from build123d import *

# Parameters (mm, degrees)
SKETCH1_W           = 20
SKETCH1_H           = 5
BOSS_EXTRUDE1_DEPTH = 4
BOSS_EXTRUDE2_DEPTH = 2
CHAMFER1_SIZE       = 0.5
CHAMFER2_SIZE       = 1
CHAMFER3_SIZE       = 1
CHAMFER3_SIZE2      = 0.707106781
FILLET5_R           = 1


with BuildPart() as part:
    # Sketch1 → Boss-Extrude1 (new body)
    with BuildSketch(Plane.XY):
        Polygon((-15, 7.5), (-15, -7.5), (-10, -2.5), (-10, 2.5), align=None)
        Rectangle(SKETCH1_W, SKETCH1_H)
        Polygon((10, 2.5), (15, 7.5), (15, -7.5), (10, -2.5), align=None)
    extrude(amount=BOSS_EXTRUDE1_DEPTH)

    # Sketch4 → Boss-Extrude2 (add, symmetric)
    with BuildSketch(Plane(origin=(0, 0, 0), x_dir=(1, 0, 0), z_dir=(0, 1, 0))):
        Polygon((3.5, 0), (-8.5, 7), (-8.5, 5), (-3.5, 0), align=None)
    extrude(amount=BOSS_EXTRUDE2_DEPTH, both=True)

    # Chamfer1
    chamfer1_edges = [part.edges().sort_by_distance(p)[0] for p in [
        (-12.5, -5, 4),
        (0, -2.5, 4),
        (12.5, -5, 4),
        (15, 0, 4),
        (12.5, 5, 4),
        (0, 2.5, 4),
        (-12.5, 5, 4),
        (-15, 0, 4),
    ]]
    chamfer(chamfer1_edges, length=CHAMFER1_SIZE)

    # Chamfer2
    # the kernel refuses this chamfer: 1 mm, written as the material it takes off along each edge
    with BuildSketch(Plane(origin=(16.81845448, -9.31845448, 0), x_dir=(0.7071067811865414, 0.7071067811865538, 0), z_dir=(-0.7071067811865538, 0.7071067811865415, 0))) as chamfer2_piece_1_section:
        Polygon((CHAMFER2_SIZE, 0), (0, -CHAMFER2_SIZE), (0, 0), align=None)
    chamfer2_piece_1 = extrude(amount=12.214433788, mode=Mode.PRIVATE)
    chamfer2_piece_1 = split(chamfer2_piece_1, bisect_by=Plane(origin=(16.81845448, -5.40922724, 3.90922724), z_dir=(0, -0.7071067811865476, -0.7071067811865476)), keep=Keep.TOP, mode=Mode.PRIVATE)
    add(chamfer2_piece_1, mode=Mode.SUBTRACT)
    with BuildSketch(Plane(origin=(15, 10.071682988, 0), x_dir=(-1, 0, 0), z_dir=(0, -1, 0)), Plane(origin=(-15, 10.071682988, 0), x_dir=(0, 0, 1), z_dir=(0, -1, 0))) as chamfer2_piece_2:
        Polygon((CHAMFER2_SIZE, 0), (0, -CHAMFER2_SIZE), (0, 0), align=None)
    extrude(amount=20.143365976, mode=Mode.SUBTRACT)
    with BuildSketch(Plane(origin=(8.18154552, 0.68154552, 0), x_dir=(0.707106781186537, -0.7071067811865581, 0), z_dir=(0.7071067811865581, 0.707106781186537, 0))) as chamfer2_piece_3_section:
        Polygon((CHAMFER2_SIZE, 0), (0, -CHAMFER2_SIZE), (0, 0), align=None)
    chamfer2_piece_3 = extrude(amount=12.214433788, mode=Mode.PRIVATE)
    chamfer2_piece_3 = split(chamfer2_piece_3, bisect_by=Plane(origin=(8.18154552, 1.09077276, -0.40922724), z_dir=(0, 0.7071067811865476, -0.7071067811865476)), keep=Keep.TOP, mode=Mode.PRIVATE)
    add(chamfer2_piece_3, mode=Mode.SUBTRACT)
    with BuildSketch(Plane(origin=(12.571682988, 2.5, 0), x_dir=(0, -1, 0), z_dir=(-1, 0, 0))) as chamfer2_piece_4_section:
        Polygon((CHAMFER2_SIZE, 0), (0, CHAMFER2_SIZE), (0, 0), align=None)
    chamfer2_piece_4 = extrude(amount=25.143365976, mode=Mode.PRIVATE)
    chamfer2_piece_4 = split(chamfer2_piece_4, bisect_by=Plane(origin=(10.268509587, 2.5, 3.948297259), z_dir=(0.5038710255240867, 0, -0.8637789008984332)), keep=Keep.TOP, mode=Mode.PRIVATE)
    chamfer2_piece_4 = split(chamfer2_piece_4, bisect_by=Plane(origin=(12.282315632, 2.789367356, -0.40922724), z_dir=(-0.4999999999999927, 0.5000000000000075, -0.7071067811865475)), keep=Keep.TOP, mode=Mode.PRIVATE)
    add(chamfer2_piece_4, mode=Mode.SUBTRACT)
    with BuildSketch(Plane(origin=(12.571682988, 2.5, 0), x_dir=(0, -1, 0), z_dir=(-1, 0, 0))) as chamfer2_piece_5_section:
        Polygon((CHAMFER2_SIZE, 0), (0, CHAMFER2_SIZE), (0, 0), align=None)
    chamfer2_piece_5 = extrude(amount=25.143365976, mode=Mode.PRIVATE)
    chamfer2_piece_5 = split(chamfer2_piece_5, bisect_by=Plane(origin=(12.571682988, 2, 0), z_dir=(0, 1, 0)), keep=Keep.TOP, mode=Mode.PRIVATE)
    chamfer2_piece_5 = split(chamfer2_piece_5, bisect_by=Plane(origin=(12.282315632, 2.789367356, -0.40922724), z_dir=(-0.4999999999999927, 0.5000000000000075, -0.7071067811865475)), keep=Keep.TOP, mode=Mode.PRIVATE)
    chamfer2_piece_5 = split(chamfer2_piece_5, bisect_by=Plane(origin=(6.57520885, -3.496474138, 8.480295052), z_dir=(0.49999999999999395, 0.500000000000006, -0.7071067811865475)), keep=Keep.TOP, mode=Mode.PRIVATE)
    add(chamfer2_piece_5, mode=Mode.SUBTRACT)
    with BuildSketch(Plane(origin=(12.571682988, 2.5, 0), x_dir=(0, -1, 0), z_dir=(-1, 0, 0))) as chamfer2_piece_6_section:
        Polygon((CHAMFER2_SIZE, 0), (0, CHAMFER2_SIZE), (0, 0), align=None)
    chamfer2_piece_6 = extrude(amount=25.143365976, mode=Mode.PRIVATE)
    chamfer2_piece_6 = split(chamfer2_piece_6, bisect_by=Plane(origin=(4.535841494, 2.5, 8.035841494), z_dir=(-0.7071067811865487, 0, 0.7071067811865464)), keep=Keep.TOP, mode=Mode.PRIVATE)
    chamfer2_piece_6 = split(chamfer2_piece_6, bisect_by=Plane(origin=(6.57520885, -3.496474138, 8.480295052), z_dir=(0.49999999999999395, 0.500000000000006, -0.7071067811865475)), keep=Keep.TOP, mode=Mode.PRIVATE)
    add(chamfer2_piece_6, mode=Mode.SUBTRACT)
    with BuildSketch(Plane(origin=(-12.571682988, -2.5, 0), x_dir=(0, 1, 0), z_dir=(1, 0, 0))) as chamfer2_piece_7_section:
        Polygon((CHAMFER2_SIZE, 0), (0, CHAMFER2_SIZE), (0, 0), align=None)
    chamfer2_piece_7 = extrude(amount=25.143365976, mode=Mode.PRIVATE)
    chamfer2_piece_7 = split(chamfer2_piece_7, bisect_by=Plane(origin=(-8.035841494, -2.5, -4.535841494), z_dir=(-0.7071067811865487, 0, 0.7071067811865464)), keep=Keep.TOP, mode=Mode.PRIVATE)
    chamfer2_piece_7 = split(chamfer2_piece_7, bisect_by=Plane(origin=(-12.282315632, -2.789367356, -0.40922724), z_dir=(0.499999999999994, -0.5000000000000063, -0.7071067811865475)), keep=Keep.TOP, mode=Mode.PRIVATE)
    add(chamfer2_piece_7, mode=Mode.SUBTRACT)
    with BuildSketch(Plane(origin=(-12.571682988, -2.5, 0), x_dir=(0, 1, 0), z_dir=(1, 0, 0))) as chamfer2_piece_8_section:
        Polygon((CHAMFER2_SIZE, 0), (0, CHAMFER2_SIZE), (0, 0), align=None)
    chamfer2_piece_8 = extrude(amount=25.143365976, mode=Mode.PRIVATE)
    chamfer2_piece_8 = split(chamfer2_piece_8, bisect_by=Plane(origin=(-12.571682988, -2, 0), z_dir=(0, -1, 0)), keep=Keep.TOP, mode=Mode.PRIVATE)
    chamfer2_piece_8 = split(chamfer2_piece_8, bisect_by=Plane(origin=(-12.282315632, -2.789367356, -0.40922724), z_dir=(0.499999999999994, -0.5000000000000063, -0.7071067811865475)), keep=Keep.TOP, mode=Mode.PRIVATE)
    chamfer2_piece_8 = split(chamfer2_piece_8, bisect_by=Plane(origin=(-6.57520885, 3.496474138, 8.480295052), z_dir=(-0.49999999999999584, -0.5000000000000047, -0.7071067811865475)), keep=Keep.TOP, mode=Mode.PRIVATE)
    add(chamfer2_piece_8, mode=Mode.SUBTRACT)
    with BuildSketch(Plane(origin=(-12.571682988, -2.5, 0), x_dir=(0, 1, 0), z_dir=(1, 0, 0))) as chamfer2_piece_9_section:
        Polygon((CHAMFER2_SIZE, 0), (0, CHAMFER2_SIZE), (0, 0), align=None)
    chamfer2_piece_9 = extrude(amount=25.143365976, mode=Mode.PRIVATE)
    chamfer2_piece_9 = split(chamfer2_piece_9, bisect_by=Plane(origin=(-8.491307514, -2.5, -6.994929383), z_dir=(0.5038710255240867, 0, -0.8637789008984332)), keep=Keep.TOP, mode=Mode.PRIVATE)
    chamfer2_piece_9 = split(chamfer2_piece_9, bisect_by=Plane(origin=(-6.57520885, 3.496474138, 8.480295052), z_dir=(-0.49999999999999584, -0.5000000000000047, -0.7071067811865475)), keep=Keep.TOP, mode=Mode.PRIVATE)
    add(chamfer2_piece_9, mode=Mode.SUBTRACT)
    with BuildSketch(Plane(origin=(-16.81845448, -9.31845448, 0), x_dir=(-0.7071067811865389, 0.7071067811865562, 0), z_dir=(0.7071067811865562, 0.7071067811865389, 0))) as chamfer2_piece_10_section:
        Polygon((CHAMFER2_SIZE, 0), (0, CHAMFER2_SIZE), (0, 0), align=None)
    chamfer2_piece_10 = extrude(amount=12.214433788, mode=Mode.PRIVATE)
    chamfer2_piece_10 = split(chamfer2_piece_10, bisect_by=Plane(origin=(-16.81845448, -5.40922724, 3.90922724), z_dir=(0, -0.7071067811865476, -0.7071067811865476)), keep=Keep.TOP, mode=Mode.PRIVATE)
    add(chamfer2_piece_10, mode=Mode.SUBTRACT)
    with BuildSketch(Plane(origin=(-8.18154552, 0.68154552, 0), x_dir=(0, 0, 1), z_dir=(-0.707106781186556, 0.707106781186539, 0))) as chamfer2_piece_11_section:
        Polygon((CHAMFER2_SIZE, 0), (0, -CHAMFER2_SIZE), (0, 0), align=None)
    chamfer2_piece_11 = extrude(amount=12.214433788, mode=Mode.PRIVATE)
    chamfer2_piece_11 = split(chamfer2_piece_11, bisect_by=Plane(origin=(-8.18154552, 1.09077276, -0.40922724), z_dir=(0, 0.7071067811865476, -0.7071067811865476)), keep=Keep.TOP, mode=Mode.PRIVATE)
    add(chamfer2_piece_11, mode=Mode.SUBTRACT)

    # Chamfer3
    chamfer3_edges = [part.edges().sort_by_distance(p)[0] for p in [
        (-3.5, 0, 0),
    ]]
    chamfer3_side = [part.faces().sort_by_distance(p)[0] for p in [
        (-5.967078189, 0, -2.467078189),
    ]]
    chamfer(chamfer3_edges, length=CHAMFER3_SIZE, length2=CHAMFER3_SIZE2, reference=chamfer3_side[0])

    # Fillet5
    # the kernel refuses this fillet: 1 mm, written as the material it takes off along each edge
    with BuildSketch(Plane(origin=(-8.5, -6.352592498, -7), x_dir=(0, 0, 1), z_dir=(0, 1, 0))) as fillet5_piece_1:
        with BuildLine():
            CenterArc((FILLET5_R * 1.74103699912, FILLET5_R), FILLET5_R, 149.743562836, 120.256437164)
            Line((FILLET5_R * 0.877258098223, FILLET5_R * 1.50387102552), (0, 0))
            Line((0, 0), (FILLET5_R * 1.74103699912, 0))
        make_face()
    extrude(amount=12.705184996, mode=Mode.SUBTRACT)
    with BuildSketch(Plane(origin=(-8.5, -3.035533906, -5), x_dir=(0, 0, -1), z_dir=(0, 1, 0))) as fillet5_piece_2:
        with BuildLine():
            CenterArc((FILLET5_R * 0.414213562373, -FILLET5_R), FILLET5_R, 90, 45)
            Line((-FILLET5_R * 0.292893218813, -FILLET5_R * 0.292893218813), (0, 0))
            Line((0, 0), (FILLET5_R * 0.414213562373, 0))
        make_face()
    extrude(amount=6.071067812, mode=Mode.SUBTRACT)


solid = part.part
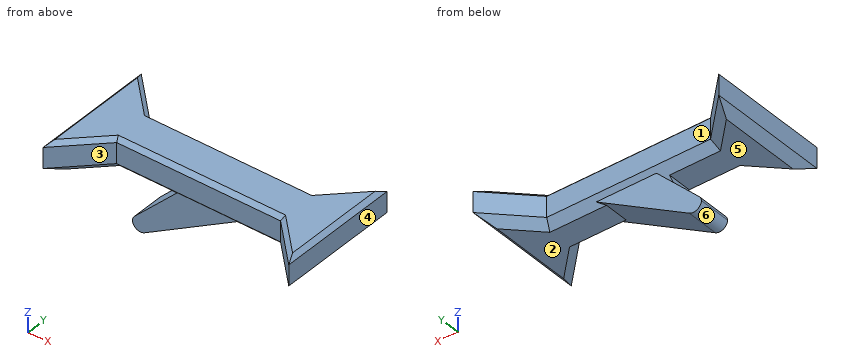
Geometry check sheet. Reference: the model listing, model coordinates, mm. Face numbers are marked on the shaded views. A direction names the side the tool comes from. Give positions to 0.01 mm unless a question says otherwise; leave off trailing zeros. Write each loop counter-clockwise with the first axis right and the second up, starting at its lowest first coordinate (ties: lowest second). Pieces come first, ordered by that corner, then holes. Notation, with made-up numbers: M 39,13.25 L 81,13.25 A31 cw 81,40.25 Z; hole C 45.25,42 d1. An arc over 180 degrees is marked long. Answer as CSV lines item,"result". Start each with the question number.
Q1. Section check C-C, the plane y = 3. Record the cut outline in (x, z), then the cut area to 3 significant figures.
Q2. Section check A-A, the plane x = -5.5. Record the cut outline in (y, z), then the cut area to 4 significant figures.
Q3. Release check for a two-part mould opening along Z. For the marked faces 4, 5 and 6 record: pulls with the +Z half, pulls with the -Z half, needs draft (parallel to the pull), parting line crosses it, or undercut.
Q4. Section check B-B, the plane z = 2.75. Record the cut outline in (x, y), then the cut area to 3 significant figures.
Q5. Section check D-D, the plane x = 5. Record the cut outline in (y, z).
Q6. Tool access check on the marked faces 1, 2 and 3. Record the directions out of +Z, -Z, +X, -X, +Y, -Y that give a thin tool (end or side, any length) a straight path to the whole face; none if there is none.
Q7. Material ranges on L1, parallel to Y at x = -6.5, z = -4; L2, parallel to Y at x = 3.5, z = 1.75; L3, parallel to X at y = -4, z = 0.75, recorded low to high.
Q8. Go/stop test with flat-tipped pins: pin 1 (5 mm diameter, centred on x = 3, z = 0, fed in from +Y); pin 2 (0.8 mm diameter, centred on x = -2, z = 2.5, fed in from -Y); pin 3 (5 mm diameter, centred on x = 11.5, y = 3.5, fed in from -Z). Record where each tip stops, or that it passes through.
Geometry says:
1,outline,"M -15,1 L -14,0 L -11.91,0 L -10.5,1 L -10.5,3.5 L -11.21,4 L -14.5,4 L -15,3.5 Z; M 10.5,1 L 11.91,0 L 14,0 L 15,1 L 15,3.5 L 14.5,4 L 11.21,4 L 10.5,3.5 Z"
1,area,"33.0 mm^2"
2,outline,"M -2.5,1 L -1.5,0 L 1.5,0 L 2.5,1 L 2.5,3.5 L 2,4 L -2,4 L -2.5,3.5 Z; M -2,-5.25 L 2,-5.25 L 2,-2 L -2,-2 Z"
2,area,"31.75 mm^2"
3,face 4,"needs draft"
3,face 5,"undercut"
3,face 6,"pulls with the -Z half"
4,outline,"M -15,-7.5 L -10,-2.5 L 10,-2.5 L 15,-7.5 L 15,7.5 L 10,2.5 L -10,2.5 L -15,7.5 Z"
4,area,"200 mm^2"
5,outline,"M -2.5,1 L -1.5,0 L 1.5,0 L 2.5,1 L 2.5,3.5 L 2,4 L -2,4 L -2.5,3.5 Z"
6,face 1,"+Z, -Z, +Y"
6,face 2,"-Z, +X, +Y, -Y"
6,face 3,"+Z, -Z, -Y"
7,L1,"-2 to 2"
7,L2,"-2.5 to 2.5"
7,L3,"-14.75 to -11.85, 11.85 to 14.75"
8,pin 1,"y = 2.5"
8,pin 2,"y = -2.5"
8,pin 3,"z = 0"
